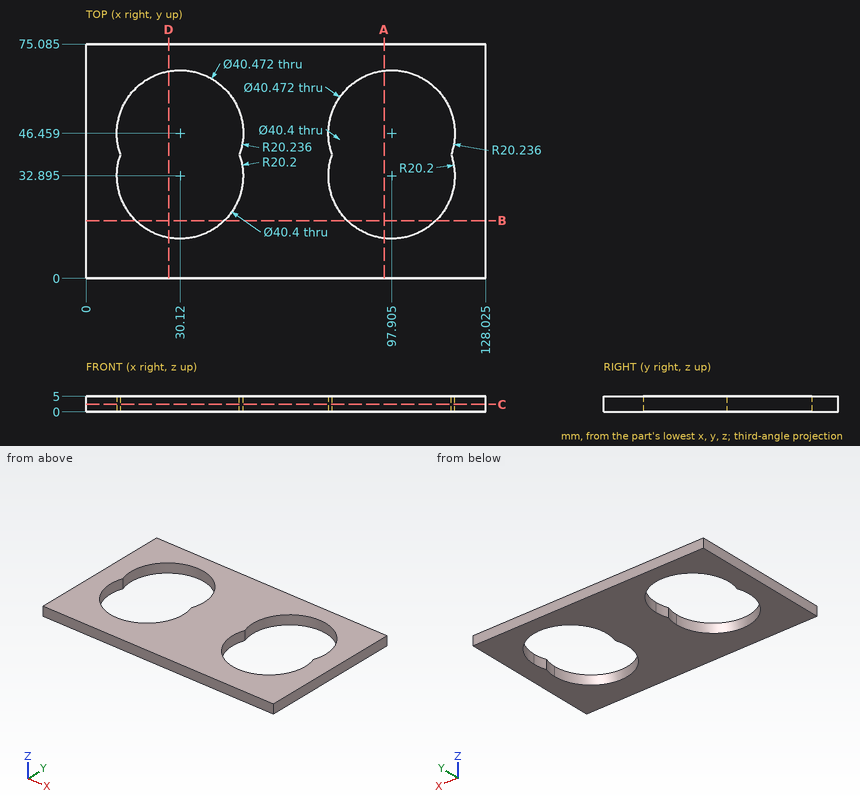
Geometry check sheet. Reference: drawing and pictorial views, mm from the part's lowest x, y, z. Coordinates: 2 decimals unless noted, no trailing zeros. Write each loop counter-clockwise with the first axis right and the second up, starting at its lowest first coordinate (ties: lowest second). Pieces come first, ordered by that corner, then holes. Notation, with made-up numbers: (3.5, 26) - (32.5, 26) arc R29 ccw to (32.5, 60) - close; hole circle Ø5 at (4, 8.25). An arc over 180 degrees is marked (long way). One line per question, with ' | ' between items. Start each with the question number.
1. Section check C-C (z = 2.4). Enter the section's corners in (x, y) (1 decimal).
2. Material ranges on line 1 along X through (y, z) = (45.5, 4.55) (1 decimal); line 2 along X through (y, z) = (34.5, 2.4) (1 decimal); line 3 along Y through (x, z) = (89, 3.7) (1 decimal), recorded low to high.
3. Section check B-B (y = 18.5). Enter the section's corners in (x, z) (1 decimal), plus the area to 3 significant figures.
4. Section check D-D (x = 26.5). Enter the section's corners in (y, z) (1 decimal).
5. Section check A-A (x = 95.5). Enter the section's corners in (y, z) (1 decimal).
Computed values:
1) outline: (0, 0) - (128, 0) - (128, 75.1) - (0, 75.1) - close; hole (11.1, 39.6) arc R20.2 ccw (long way) to (49.2, 39.6) arc R20.2 ccw (long way) to start; hole (78.9, 39.6) arc R20.2 ccw (long way) to (117, 39.6) arc R20.2 ccw (long way) to start
2) line 1: 0 to 9.9, 50.3 to 77.7, 118.1 to 128 | line 2: 0 to 10, 50.3 to 77.8, 118 to 128 | line 3: 0 to 14.8, 64.6 to 75.1
3) outline: (0, 0) - (15.9, 0) - (15.9, 5) - (0, 5) - close; (44.3, 0) - (83.7, 0) - (83.7, 5) - (44.3, 5) - close; (112.1, 0) - (128, 0) - (128, 5) - (112.1, 5) - close | area: 357 mm²
4) outline: (0, 0) - (13, 0) - (13, 5) - (0, 5) - close; (66.4, 0) - (75.1, 0) - (75.1, 5) - (66.4, 5) - close
5) outline: (0, 0) - (12.8, 0) - (12.8, 5) - (0, 5) - close; (66.6, 0) - (75.1, 0) - (75.1, 5) - (66.6, 5) - close
